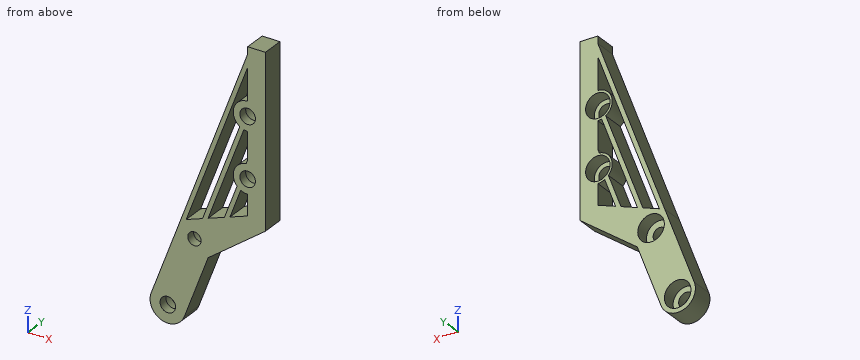
from build123d import *

# Parameters (mm, degrees)
SKIZZE1_R                       = 1.75
SKIZZE1_R_2                     = 1.5
AUFSATZ_LINEAR_AUSTRAGEN1_DEPTH = 5
AUFSATZ_LINEAR_AUSTRAGEN2_DEPTH = 5
SKIZZE4_R                       = 3.25
AUFSATZ_LINEAR_AUSTRAGEN3_DEPTH = 5
SKIZZE5_R                       = 1.75
SCHNITT_LINEAR_AUSTRAGEN2_DEPTH = 5
SKIZZE3_R                       = 3
SKIZZE3_R_2                     = 2.75
SCHNITT_LINEAR_AUSTRAGEN1_DEPTH = 3
SCHNITT_LINEAR_AUSTRAGEN3_DEPTH = 5


with BuildPart() as part:
    # Skizze1 → Aufsatz-Linear austragen1 (new body)
    with BuildSketch(Plane(origin=(0, 0, 0), x_dir=(1, 0, 0), z_dir=(0, 1, 0))):
        with BuildLine():
            Line((-3.74531671, -1.404493766), (2.906480569, -19.142619845))
            Line((2.906480569, -19.142619845), (18, -24.533162499))
            Line((18, -24.533162499), (18, -61))
            Line((18, -61), (22, -61))
            Line((22, -61), (22, -17.466837501))
            Line((22, -17.466837501), (9.093519431, -12.857380155))
            Line((9.093519431, -12.857380155), (3.74531671, 1.404493766))
            ThreePointArc((3.74531671, 1.404493766), (-1.404493766, 3.74531671), (-3.74531671, -1.404493766))
        make_face()
        Circle(SKIZZE1_R, mode=Mode.SUBTRACT)
        with Locations((6, -16)):
            Circle(SKIZZE1_R_2, mode=Mode.SUBTRACT)
    extrude(amount=AUFSATZ_LINEAR_AUSTRAGEN1_DEPTH)

    # Skizze2 → Aufsatz-Linear austragen2 (add)
    with BuildSketch(Plane(origin=(0, 5, 0), x_dir=(1, 0, 0), z_dir=(0, 1, 0))):
        Polygon((2.906480569, -19.142619845), (18, -59.392004994), (18, -56.544003745), (4.139635749, -19.58303241), align=None)
        Polygon((7.839101288, -20.904270102), (18, -48), (18, -45.151998752), (9.072256468, -21.344682666), align=None)
        Polygon((12.771722007, -22.665920359), (18, -36.607995006), (18, -33.759993758), (14.004877187, -23.106332923), align=None)
    extrude(amount=-AUFSATZ_LINEAR_AUSTRAGEN2_DEPTH)

    # Skizze4 → Aufsatz-Linear austragen3 (add)
    with BuildSketch(Plane(origin=(0, 5, 0), x_dir=(1, 0, 0), z_dir=(0, 1, 0))):
        with Locations((18, -32.466837501)):
            Circle(SKIZZE4_R)
        with Locations((18, -46)):
            Circle(SKIZZE4_R)
    extrude(amount=-AUFSATZ_LINEAR_AUSTRAGEN3_DEPTH)

    # Skizze5 → Schnitt-Linear austragen2 (cut)
    with BuildSketch(Plane(origin=(0, 5, 0), x_dir=(1, 0, 0), z_dir=(0, 1, 0))):
        with Locations((18, -32.466837501)):
            Circle(SKIZZE5_R)
        with Locations((18, -46)):
            Circle(SKIZZE5_R)
    extrude(amount=-SCHNITT_LINEAR_AUSTRAGEN2_DEPTH, mode=Mode.SUBTRACT)

    # Skizze3 → Schnitt-Linear austragen1 (cut)
    with BuildSketch(Plane(origin=(0, 5, 0), x_dir=(1, 0, 0), z_dir=(0, 1, 0))):
        Circle(SKIZZE3_R)
        with Locations((6, -16)):
            Circle(SKIZZE3_R)
        with Locations((18, -32.466837501)):
            Circle(SKIZZE3_R_2)
        with Locations((18, -46)):
            Circle(SKIZZE3_R_2)
    extrude(amount=-SCHNITT_LINEAR_AUSTRAGEN1_DEPTH, mode=Mode.SUBTRACT)

    # Skizze6 → Schnitt-Linear austragen3 (cut)
    with BuildSketch(Plane(origin=(0, 5, 0), x_dir=(1, 0, 0), z_dir=(0, 1, 0))):
        Polygon((9.093519431, -12.857380155), (22, -22.466837501), (22, -17.466837501), align=None)
    extrude(amount=-SCHNITT_LINEAR_AUSTRAGEN3_DEPTH, mode=Mode.SUBTRACT)


solid = part.part
Input: part model. Units: mm. Frame: model coordinates. Coordinates: 2 decimals unless noted, no trailing zeros. Order: outer loops, then holes, each group sorted by start corner. A loop starts at its lowest first (then second) coordinate and runs counter-clockwise, first axis right, second up. Notation, with made-up numbers: M 61.5,13 L 68.5,13 A21 ccw 68.5,36 Z; hole C 47.5,60 d6. An arc over 180 degrees is marked long. Answer as CSV lines item,"result".
1. Section B-B (x = 6). Return the cut outline in (y, z), then the cut area to 3 significant figures.
Reported:
outline,"M 0,4.61 L 5,4.61 L 5,13 L 2,13 L 2,14.5 L 0,14.5 Z; M 0,17.5 L 2,17.5 L 2,19 L 5,19 L 5,20.25 L 0,20.25 Z; M 0,24.54 L 5,24.54 L 5,27.39 L 0,27.39 Z"
area,"68.4 mm2"
2. First-contact query: P1, Ø2, axis at x = 0, z = 0, coming from the +Y side; P2, Ø2, axis at x = 13.5, y = 4, coming from the -Z side; P3, Ø5.5, axis at x = 6, z = 16, coming from the +Y side. Flat tips, straight axial feed; report the tip coordinate or a pass-through.
Reported:
P1,"through"
P2,"z = 15.39"
P3,"y = 2"
3. Section C-C (y = 1.1). Return the cut outline in (x, z).
Reported:
outline,"M -3.75,1.4 A4 ccw 3.75,-1.4 L 9.09,12.86 L 22,22.47 L 22,61 L 18,61 L 18,59.39 Z; hole C 0,0 d3.5; hole M 4.14,19.58 L 7.84,20.9 L 16.23,43.28 A3.25 cw 18,49.25 L 18,56.54 Z; hole C 6,16 d3; hole M 9.07,21.34 L 12.77,22.67 L 15.62,30.26 A3.25 cw 17.66,35.7 L 18,36.61 L 18,42.75 A3.25 cw 17.14,42.87 Z; hole M 14,23.11 L 18,24.53 L 18,29.22 A3.25 cw 16.44,29.61 Z; hole C 18,32.47 d3.5; hole C 18,46 d3.5"
4. Section A-A (z = 53). Return the cut outline in (x, y).
Reported:
outline,"M 15.6,0 L 16.67,0 L 16.67,5 L 15.6,5 Z; M 18,0 L 22,0 L 22,5 L 18,5 Z"
5. Section D-D (z = 38.5). Return the cut outline in (x, y), then the cut area to 3 significant figures.
Reported:
outline,"M 10.17,0 L 11.23,0 L 11.23,5 L 10.17,5 Z; M 14.44,0 L 15.51,0 L 15.51,5 L 14.44,5 Z; M 18,0 L 22,0 L 22,5 L 18,5 Z"
area,"30.7 mm2"
6. Material intervals for line 1 (X direction, y = 4.6, z = 23) (3 decimals); line 2 (Z direction, x = 20, y = 3.15); line 3 (Z direction, x = 19.25, y = 0.3), sorted ascending. Write a range as from..to.
Reported:
line 1,"4.353..5.421, 8.625..9.693, 12.897..22"
line 2,"20.98..30.58, 34.35..44.11, 47.89..61"
line 3,"20.42..31.24, 33.69..44.78, 47.22..61"
